Check sheet for the drawn part. Datum: minimum x, y, z corner. Units: mm. A direction names the side the tool comes from. Give positions to 0.01 mm unless a question says otherwise; leave off trailing zeros. Order: outer loops, then holes, each group sorted by start corner. A loop starts at its lowest first (then second) coordinate and runs counter-clockwise, first axis right, second up. Notation, with made-up numbers: M 54,67 L 58,67 A28 cw 58,92 Z; hole C -10.5,3.5 d3. An arc over 180 degrees is marked long. One line per question, with ' | ' between items. Start each with the question number.
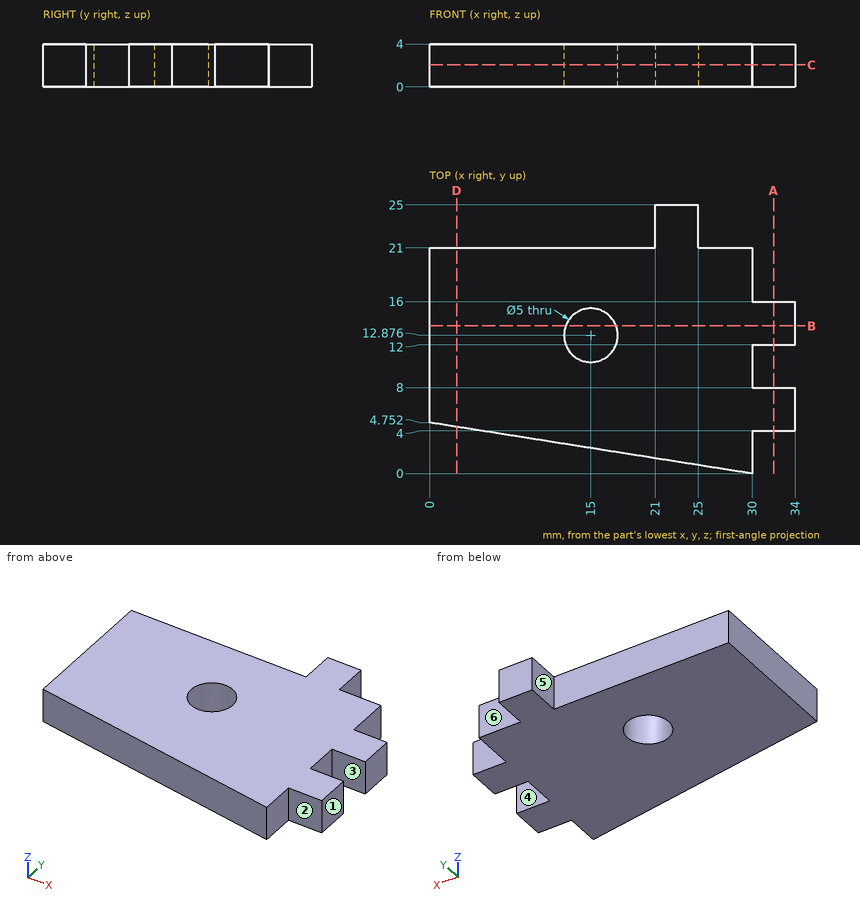
Item 1: Go/stop test with flat-tipped pins: P1, Ø2, axis at y = 23.5, z = 1, coming from the -X side; P2, Ø3, axis at x = 15, y = 12.88, coming from the +Z side; P3, Ø2, axis at y = 23.5, z = 2, coming from the +X side; P4, Ø2, axis at x = 31.5, z = 2, coming from the -Y side. Record where each tip stops, or that it passes through.
Item 2: Set-up check for the marked faces 4, 5 and 6: record each of +Z, -Z, +X, -X, +Y, -Y from which the full face is reachable in a straight line by a thin tool's end or side.
Item 3: Section check A-A, the plane x = 32. Record the cut outline in (y, z), then the cut area to 3 significant figures.
Item 4: Section check D-D, the plane x = 2.5. Record the cut outline in (y, z) (1 decimal).
Item 5: Section check B-B, the plane y = 13.75. Record the cut outline in (x, z), then the cut area to 3 significant figures.
Item 6: Section check C-C, the plane z = 2.05. Record the cut outline in (x, y) (1 decimal).
Item 7: Draft check along Y on the marked faces 1, 2 and 3. Enter one of: released by +Y, released by -Y, zero draft, split by the parting line, or undercut.
Item 8: Scan lines: probe 1 along X at (y, z) = (12.75, 2.7); probe 2 along Y at (x, z) = (31, 2.25); probe 3 along X at (y, z) = (22.25, 3.6). Record each from-to range of solid material in increasing order. Write a range as [from, to].
Reported:
1) P1: stops at x = 21 | P2: passes through | P3: stops at x = 25 | P4: stops at y = 4
2) face 4: +Z, -Z, +X | face 5: +Z, -Z, -X, +Y | face 6: +Z, -Z, +X, +Y
3) outline: M 4,0 L 8,0 L 8,4 L 4,4 Z; M 12,0 L 16,0 L 16,4 L 12,4 Z | area: 32.0 mm^2
4) outline: M 4.4,0 L 21,0 L 21,4 L 4.4,4 Z
5) outline: M 0,0 L 12.66,0 L 12.66,4 L 0,4 Z; M 17.34,0 L 34,0 L 34,4 L 17.34,4 Z | area: 117 mm^2
6) outline: M 0,4.8 L 30,0 L 30,4 L 34,4 L 34,8 L 30,8 L 30,12 L 34,12 L 34,16 L 30,16 L 30,21 L 25,21 L 25,25 L 21,25 L 21,21 L 0,21 Z; hole C 15,12.9 d5
7) face 1: zero draft | face 2: released by -Y | face 3: undercut
8) probe 1: x = [0, 12.5], [17.5, 34] | probe 2: y = [4, 8], [12, 16] | probe 3: x = [21, 25]
